Part model, mm, in its own coordinate system. Face numbers are marked on the shaded views. Give positions to 0.01 mm unless a question says otherwise; leave off trailing zeros. Write each loop counter-clockwise with the first axis right and the second up, starting at its lowest first coordinate (ties: lowest second). Pieces come first, ordered by that corner, then holes. Notation, with made-up numbers: M -38,-2 L -21,-2 A34 cw -21,37 Z; hole C 15.5,30.5 d10. An arc over 180 degrees is marked long. Write item = value, one per line. Start each with the question number.
Autodesk Inventor part; units mm, degrees
ref_plane "YZ Plane" through (0, 0, 0) normal (1, 0, 0) x (0, 1, 0)
ref_plane "XZ Plane" through (0, 0, 0) normal (0, 1, 0) x (-1, 0, 0)
ref_plane "XY Plane" through (0, 0, 0) normal (0, 0, 1) x (1, 0, 0)
sketch "Sketch1" plane through (0, 0, 0) normal (0, 1, 0) x (-1, 0, 0)
  line L0 (0, 0) -> (50.175, 0)
  line L1 (50.175, 0) -> (50.175, -77.485)
  line L2 (50.175, -77.485) -> (0, -77.485)
  line L3 (0, -77.485) -> (0, 0)
  circle A0 centre (48.265, -1.91) radius 2.1
  circle A1 centre (48.265, -75.575) radius 2.1
  circle A2 centre (1.91, -1.91) radius 2.1
  circle A3 centre (1.91, -75.575) radius 2.1
  line L4 (50.175, 0) -> (53.985, 0)
  line L5 (53.985, 0) -> (53.985, -77.675)
  line L6 (53.985, -77.675) -> (50.175, -77.675)
  line L7 (50.175, -77.675) -> (50.175, 0)
  line L8 (0, 0) -> (-3.81, 0)
  line L9 (-3.81, 0) -> (-3.81, -77.675)
  line L10 (-3.81, -77.675) -> (0, -77.675)
  line L11 (0, -77.675) -> (0, 0)
  line L12 (53.985, -77.675) -> (-3.81, -77.675)
  line L13 (-3.81, -77.675) -> (-3.81, -81.485)
  line L14 (-3.81, -81.485) -> (53.985, -81.485)
  line L15 (53.985, -81.485) -> (53.985, -77.675)
  line L16 (-3.81, 0) -> (53.985, 0)
  line L17 (53.985, 0) -> (53.985, 3.81)
  line L18 (53.985, 3.81) -> (-3.81, 3.81)
  line L19 (-3.81, 3.81) -> (-3.81, 0)
  point P0 (0, -77.485)
  point P1 (0, -76.4479)
  point P2 (0, -74.7021)
  point P3 (0, -2.7829)
  point P4 (0, -1.0371)
  dimension "d0" = 77.485
  dimension "d1" = 50.175
  dimension "d3" = 4.2
  dimension "d4" = 4.2
  dimension "d6" = 1.91
  dimension "d7" = 1.91
  dimension "d8" = 1.91
  dimension "d9" = 4.2
  dimension "d10" = 4.2
  dimension "d11" = 1.91
  dimension "d12" = 1.91
  dimension "d13" = 1.91
  dimension "d14" = 1.91
  dimension "d15" = 1.91
  dimension "d18" = 3.81
  dimension "d19" = 3.81
  dimension "d20" = 3.81
  dimension "d21" = 3.81
extrude "Extrusion2" add sketch "Sketch1" along normal blind 6 contours L8 L19 L18 L17 L4 L0 A0 A2 | L0 A2 L3 | L3 A2 A3 L11 L10 L9 L8 | L0 A0 L1 A1 L2 A3 L3 A2 | L10 L12 L6 L15 L14 L13 | L11 L2 A3 L12 | L0 L1 A0 | A0 L1 L4 L5 L6 L7 A1 | A3 L2 L3 | A3 L2 A1 L12 | A1 L2 L7 L12 | L1 L2 A1 picked at (0.2904, -0.2904) picked at (49.8846, -0.2904) picked at (0.2904, -77.1946) picked at (49.8846, -77.1946)
sketch "Sketch2" plane through (0, 6, 0) normal (0, 1, 0) x (1, 0, 0)
  circle A0 centre (-1.91, 1.91) radius 2.1
  circle A1 centre (-48.265, 1.91) radius 2.1
  circle A2 centre (-48.265, 75.575) radius 2.1
  line L0 (3.81, -3.81) -> (3.81, 81.485)
  line L1 (3.81, 81.485) -> (-53.985, 81.485)
  line L2 (-53.985, 81.485) -> (-53.985, -3.81)
  line L3 (-53.985, -3.81) -> (3.81, -3.81)
  circle A3 centre (-1.91, 75.575) radius 2.1
  point P0 (0, 0)
sketch "Sketch3" plane through (0, 0, 0) normal (0, -1, 0) x (1, 0, 0)
  line L0 (-53.985, 3.81) -> (3.81, 3.81)
  line L1 (-53.985, 3.81) -> (3.81, 3.81)
  line L2 (3.81, 3.81) -> (3.81, 6.35)
  line L3 (3.81, 6.35) -> (-53.985, 6.35)
  line L4 (-53.985, 6.35) -> (-53.985, 3.81)
  circle A0 centre (-1.91, -1.91) radius 2.1
  circle A1 centre (-48.265, -1.91) radius 2.1
  circle A2 centre (-48.265, -75.575) radius 2.1
  line L5 (3.81, 3.81) -> (3.81, -81.485)
  line L6 (-53.985, 3.81) -> (3.81, 3.81)
  line L7 (-53.985, -81.485) -> (-53.985, 3.81)
  line L8 (3.81, -81.485) -> (-53.985, -81.485)
  circle A3 centre (-1.91, -75.575) radius 2.1
  line L9 (3.81, 6.35) -> (6.35, 6.35)
  line L10 (6.35, 6.35) -> (6.35, -81.485)
  line L11 (6.35, -81.485) -> (3.81, -81.485)
  line L12 (3.81, -81.485) -> (3.81, 6.35)
  line L13 (3.81, -81.485) -> (-53.985, -81.485)
  line L14 (-53.985, -81.485) -> (6.35, -81.485)
  line L15 (6.35, -81.485) -> (6.35, -84.025)
  line L16 (6.35, -84.025) -> (-53.985, -84.025)
  line L17 (-53.985, -84.025) -> (-53.985, -81.485)
  line L18 (-53.985, 6.35) -> (-56.525, 6.35)
  line L19 (-56.525, 6.35) -> (-56.525, -84.025)
  line L20 (-56.525, -84.025) -> (-53.985, -84.025)
  line L21 (-53.985, -84.025) -> (-53.985, 6.35)
  point P0 (0, 0)
  dimension "d24" = 2.54
  dimension "d25" = 2.54
  dimension "d26" = 2.54
  dimension "d27" = 2.54
extrude "Extrusion3" add sketch "Sketch3" against normal blind 10.16 contours L4 L3 L2 L0 | L7 L17 L20 L19 L18 L4 | L2 L9 L10 L11 L5 | L8 L11 L15 L16 L17
sketch "Sketch4" plane through (0, 6, 0) normal (0, 1, 0) x (1, 0, 0)
  point P0 (0, 0)
sketch "Sketch5" plane through (0, 6, 0) normal (0, 1, 0) x (1, 0, 0)
  circle A0 centre (-1.91, 1.91) radius 2.1
  circle A1 centre (-48.265, 1.91) radius 2.1
  circle A2 centre (-48.265, 75.575) radius 2.1
  line L0 (3.81, -3.81) -> (3.81, 81.485)
  line L1 (3.81, 81.485) -> (-53.985, 81.485)
  line L2 (-53.985, 81.485) -> (-53.985, -3.81)
  line L3 (-53.985, -3.81) -> (3.81, -3.81)
  circle A3 centre (-1.91, 75.575) radius 2.1
  line L4 (-56.525, 84.025) -> (-56.525, -6.35)
  line L5 (-53.985, -3.81) -> (-53.985, 81.485)
  line L6 (-53.985, -3.81) -> (3.81, 81.485)
  line L7 (-53.985, 81.485) -> (-53.985, -3.81)
  line L8 (-53.985, 81.485) -> (3.81, -3.81)
  line L9 (-53.985, 81.485) -> (-41.285, 81.485)
  line L10 (-41.285, 81.485) -> (-41.285, 68.785)
  line L11 (-41.285, 68.785) -> (-53.985, 68.785)
  line L12 (-53.985, 68.785) -> (-53.985, 81.485)
  line L13 (3.81, 81.485) -> (-53.985, 81.485)
  line L14 (3.81, 81.485) -> (-8.89, 81.485)
  line L15 (-8.89, 81.485) -> (-8.89, 68.785)
  line L16 (-8.89, 68.785) -> (3.81, 68.785)
  line L17 (3.81, 68.785) -> (3.81, 81.485)
  line L18 (-53.985, -3.81) -> (3.81, -3.81)
  line L19 (-53.985, -3.81) -> (-41.285, -3.81)
  line L20 (-41.285, -3.81) -> (-41.285, 8.89)
  line L21 (-41.285, 8.89) -> (-53.985, 8.89)
  line L22 (-53.985, 8.89) -> (-53.985, -3.81)
  line L23 (3.81, -3.81) -> (-8.89, -3.81)
  line L24 (-8.89, -3.81) -> (-8.89, 8.89)
  line L25 (-8.89, 8.89) -> (3.81, 8.89)
  line L26 (3.81, 8.89) -> (3.81, -3.81)
  point P0 (0, 0)
  dimension "d30" = 12.7
  dimension "d31" = 12.7
  dimension "d32" = 12.7
  dimension "d33" = 12.7
  dimension "d34" = 12.7
  dimension "d35" = 12.7
extrude "Extrusion4" cut sketch "Sketch5" against normal blind 2.54 contours L25 L24 L3 L20 L21 L6 L8 | L8 L6 L16 L0 L25 | L8 L11 L10 L1 L15 L16 L6 | L6 L21 L2 L11 L8
properties part number "PCB_BOARD_Holder_"
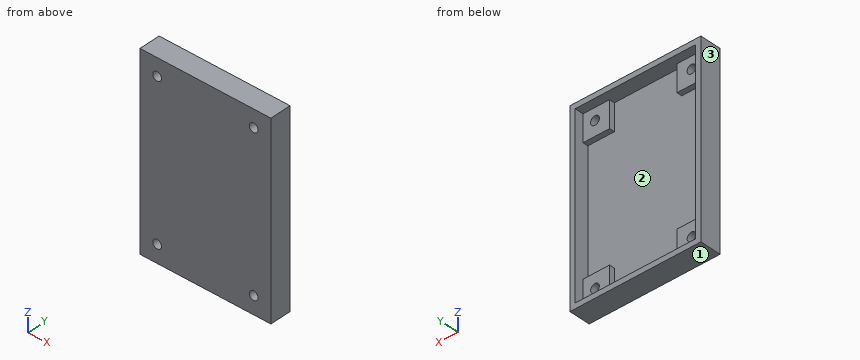
Q1. Slice it at B-B (x = -1.91). Give the cut face in (y, z) (3 decimals), and give its area (3 significant figures).
Q2. Drop flat-ended pins along their axis: P1, Ø12, axis at x = -14, z = -38.5, coming from the -Y side; P2, Ø2, axis at x = -15.5, z = -39, coming from the +Y side; P3, Ø6.5, axis at x = -47, z = -5.5, coming from the +Y side. Give the stop position or say it passes through.
Q3. Two-plate mould, pull along Z, no slides. Class the marked faces 1, 2 and 3: +Z half, -Z half, draft (parallel to the pull), parting line (faces both ways), or undercut.
Q4. Probe line 1 along X through (y, z) = (4.65, -1.91) (3 decimals); line 2 along Z through (x, y) = (-1.91, 4.85) (3 decimals); line 3 along X through (y, z) = (1.65, -1.91) (3 decimals). List the from-to ranges inside material, lowest first.
Q5. Slice it at D-D (x = -45). Give the cut face in (y, z) (3 decimals), and give its area (3 significant figures).
Q6. Slice it at C-C (z = -15.5). Give the cut face in (x, y) (3 decimals), and give its area (3 significant figures).
Q7. Slice it at A-A (z = -1.91). Give the cut face in (x, y) (3 decimals), and give its area (3 significant figures).
Working result:
q1.outline = M 0,-84.025 L 10.16,-84.025 L 10.16,-81.485 L 6,-81.485 L 6,-77.675 L 0,-77.675 Z; M 0,-73.475 L 6,-73.475 L 6,-68.785 L 3.46,-68.785 L 3.46,-8.89 L 6,-8.89 L 6,-4.01 L 0,-4.01 Z; M 0,0.19 L 6,0.19 L 6,3.81 L 10.16,3.81 L 10.16,6.35 L 0,6.35 Z
q1.area = 361 mm2
q2.P1 = 0
q2.P2 = 3.46
q2.P3 = 6
q3.face_1 = -Z half
q3.face_2 = undercut
q3.face_3 = draft
q4.line_1 = -56.525 to -50.365, -46.165 to -41.285, -8.89 to -4.01, 0.19 to 6.35
q4.line_2 = -84.025 to -77.675, -73.475 to -68.785, -8.89 to -4.01, 0.19 to 6.35
q4.line_3 = -56.525 to -50.365, -46.165 to -4.01, 0.19 to 6.35
q5.outline = M 0,-84.025 L 10.16,-84.025 L 10.16,-81.485 L 6,-81.485 L 6,-68.785 L 3.46,-68.785 L 3.46,-8.89 L 6,-8.89 L 6,3.81 L 10.16,3.81 L 10.16,6.35 L 0,6.35 Z
q5.area = 411 mm2
q6.outline = M -56.525,0 L 6.35,0 L 6.35,10.16 L 3.81,10.16 L 3.81,3.46 L -53.985,3.46 L -53.985,10.16 L -56.525,10.16 Z
q6.area = 252 mm2
q7.outline = M -56.525,0 L -50.365,0 L -50.365,6 L -53.985,6 L -53.985,10.16 L -56.525,10.16 Z; M -46.165,0 L -4.01,0 L -4.01,6 L -8.89,6 L -8.89,3.46 L -41.285,3.46 L -41.285,6 L -46.165,6 Z; M 0.19,0 L 6.35,0 L 6.35,10.16 L 3.81,10.16 L 3.81,6 L 0.19,6 Z
q7.area = 266 mm2
